Check sheet for the modelled part. Datum: model origin and axes. Units: mm. A direction names the side the tool comes from. Round coordinates to 2 decimals unless told otherwise and drop trailing zeros. Loops run counter-clockwise (first coordinate to the right, second up) from the corner with the lowest first, then second, coordinate; pieces in that order, holes last. Notation, with made-up numbers: M 0.25,38 L 15.25,38 A33 cw 15.25,70 Z; hole C 55,27.5 d6. An arc over 180 degrees is marked long. Write item = value, one per line. Start each with the question number.
(1) Mould release check, pull along Y, two halves, no side actions. Record for faces 3 (the face through (-35.983, 16.061, 4.024)), 4 (the face through (-1, -21, 7.938)), 5 (the face through (-10.407, 46.864, 3.913)): pulls with the +Y half, pulls with the -Y half, needs draft (parallel to the pull), parting line crosses it, or undercut.
(2) Go/stop test with flat-tipped pins: P1, Ø4, axis at x = -11, z = 6.5, coming from the -Y side; P2, Ø3, axis at y = 4, z = 4, coming from the +X side; P3, Ø5.5, axis at x = -32.476, y = -18.75, coming from the +Z side; P4, Ø4, axis at x = 8.5, z = 3.5, coming from the -Y side. Record where each tip stops, or that it passes through.
(3) Cross-section at B-B on z = 5. Record the boundary of the cut face in (x, y).
(4) Set-up check for faces 1 (the face through (-11, 1, 0)), 2 (the face through (0, -9.97, 3)): record each of +Z, -Z, +X, -X, +Y, -Y from which the full face is reachable in a straight line by a thin tool's end or side.
(5) Scan lines: L1, parallel to Y at x = 0, z = 2; L2, parallel to Y at x = 33, z = 0.5; L3, parallel to Y at x = -29, z = 4.25. Record each from-to range of solid material in increasing order. Write a range as from..to.
(6) Cross-section at A-A on y = 0. Record the boundary of the cut face in (x, z).
(7) Cross-section at C-C on x = 32. Record the boundary of the cut face in (y, z), plus the area to 3 significant figures.
(8) Cross-section at D-D on y = 20. Record the boundary of the cut face in (x, z), plus the area to 3 significant figures.
Autodesk Inventor part; units mm, degrees
ref_plane "YZ Plane" through (0, 0, 0) normal (1, 0, 0) x (0, 1, 0)
ref_plane "XZ Plane" through (0, 0, 0) normal (0, 1, 0) x (-1, 0, 0)
ref_plane "XY Plane" through (0, 0, 0) normal (0, 0, 1) x (1, 0, 0)
sketch "Sketch1" plane through (0, 0, 0) normal (0, 0, 1) x (1, 0, 0)
  circle A0 centre (0, 0) radius 48.006
  dimension "d0" = 96.012
extrude "Extrusion1" add sketch "Sketch1" along normal blind 7.9375
sketch "Sketch2" plane through (0, 0, 7.9375) normal (0, 0, 1) x (1, 0, 0)
  circle A0 centre (0, 37.5) radius 4.4196
  circle A1 centre (-32.476, 18.75) radius 4.4196
  circle A2 centre (-32.476, -18.75) radius 4.4196
  circle A3 centre (0, -37.5) radius 4.4196
  circle A4 centre (32.476, -18.75) radius 4.4196
  circle A5 centre (32.476, 18.75) radius 4.4196
  circle A6 centre (0, 0) radius 37.5
  dimension "d17" = 75
  dimension "d3" = 8.8392
  dimension "d7" = 360
extrude "Extrusion2" cut sketch "Sketch2" against normal through all contours A0 A6 | A6 A0 | A6 A1 | A1 A6 | A6 A5 | A5 A6 | A6 A2 | A2 A6 | A6 A4 | A4 A6 | A6 A3 | A3 A6
sketch "Sketch3" plane through (0, 0, 7.9375) normal (0, 0, 1) x (1, 0, 0)
  line L0 (-9.9695, -9.9695) -> (9.9695, -9.9695)
  line L1 (9.9695, -9.9695) -> (9.9695, 9.9695)
  line L2 (9.9695, 9.9695) -> (-9.9695, 9.9695)
  line L3 (-9.9695, 9.9695) -> (-9.9695, -9.9695)
  line L4 (-9.9695, -9.9695) -> (9.9695, 9.9695) construction
  line L5 (9.9695, -9.9695) -> (-9.9695, 9.9695) construction
  point P0 (0, 0)
  dimension "d11" = 19.939
extrude "Extrusion3" cut sketch "Sketch3" against normal through all
chamfer "Chamfer1" distance 1.5875 angle 45 4 edges at (0, 9.9695, 7.9375) (-9.9695, 0, 7.9375) (0, -9.9695, 7.9375) (9.9695, 0, 7.9375)
properties part number "Adam's Shaft plate rev 2"
Result:
q1.face_3 = undercut
q1.face_4 = needs draft
q1.face_5 = parting line crosses it
q2.P1 = -47.15
q2.P2 = 47.94
q2.P3 = through
q2.P4 = -47.56
q3.outline = C 0,0 d96.01; hole C -32.48,-18.75 d8.84; hole C -32.48,18.75 d8.84; hole M -9.97,-9.97 L 9.97,-9.97 L 9.97,9.97 L -9.97,9.97 Z; hole C 0,-37.5 d8.84; hole C 0,37.5 d8.84; hole C 32.48,-18.75 d8.84; hole C 32.48,18.75 d8.84
q4.face_1 = -Z, +X, -X, +Y, -Y
q4.face_2 = +Z, -Z
q5.L1 = -48.01..-41.92, -33.08..-9.97, 9.97..33.08, 41.92..48.01
q5.L2 = -34.87..-23.14, -14.36..14.36, 23.14..34.87
q5.L3 = -38.26..-21.48, -16.02..16.02, 21.48..38.26
q6.outline = M -48.01,0 L -9.97,0 L -9.97,6.35 L -11.56,7.94 L -48.01,7.94 Z; M 9.97,0 L 48.01,0 L 48.01,7.94 L 11.56,7.94 L 9.97,6.35 Z
q7.outline = M -35.79,0 L -23.14,0 L -23.14,7.94 L -35.79,7.94 Z; M -14.36,0 L 14.36,0 L 14.36,7.94 L -14.36,7.94 Z; M 23.14,0 L 35.79,0 L 35.79,7.94 L 23.14,7.94 Z
q7.area = 429 mm^2
q8.outline = M -43.64,0 L -36.72,0 L -36.72,7.94 L -43.64,7.94 Z; M -28.24,0 L 28.24,0 L 28.24,7.94 L -28.24,7.94 Z; M 36.72,0 L 43.64,0 L 43.64,7.94 L 36.72,7.94 Z
q8.area = 558 mm^2
